Model file for the job. Use its own axes, mm. Face numbers are marked on the shaded views. A direction names the side the tool comes from. Give positions to 0.01 mm unless a question says otherwise; leave off trailing zeros. Loops run counter-clockwise (first coordinate to the right, second up) from the corner with the lowest first, then second, coordinate; pieces in that order, holes last. Notation, with made-up numbers: (45, -3.5) - (63, -3.5) arc R19 cw to (63, 2.5) - close; hole circle Ø3 at (-39, -15). An arc over 180 degrees is marked (long way). Answer as CSV lines item,"result". Start each with the question number.
Item 1: Drill centre lines: L1, parallel to Y at x = 0, z = 2.45; L2, parallel to Y at x = -1.25, z = 1.55; L3, parallel to X at y = 6, z = 2.25. Where is each one in solid material? Low to high. Write a range as from..to.
Item 2: Tool access for the marked faces 1 and 2: list every direction of +Z, -Z, +X, -X, +Y, -Y with a clear straight run to the whole face (end or side of a thin tool).
Item 3: Saw through at C-C on z = 1.1. Give the cut face in (x, y), plus the area to 3 significant figures.
Item 4: Saw through at B-B on x = 1. Give the cut face in (y, z), plus the area to 3 significant figures.
Item 5: Pin check, flat tips, straight feed: pin 1 (7 mm diameter, centred on x = 0, y = -25, fed in from -Z); pin 2 (2 mm diameter, centred on x = -4, z = 4, fed in from +Y); pin 3 (1 mm diameter, centred on x = 5, z = 3.5, fed in from -Y). Stop position of each tip, or through.
Item 6: Pull direction Y, two halves, no side cores. Call the marked faces 3, 4, 5 and 6: pulls with the +Y half, pulls with the -Y half, needs draft (parallel to the pull), parting line crosses it, or undercut.
Item 7: Saw through at D-D on y = 24. Give the cut face in (x, z).
Item 8: Saw through at A-A on y = 8. Give the cut face in (x, z), plus the area to 3 significant figures.
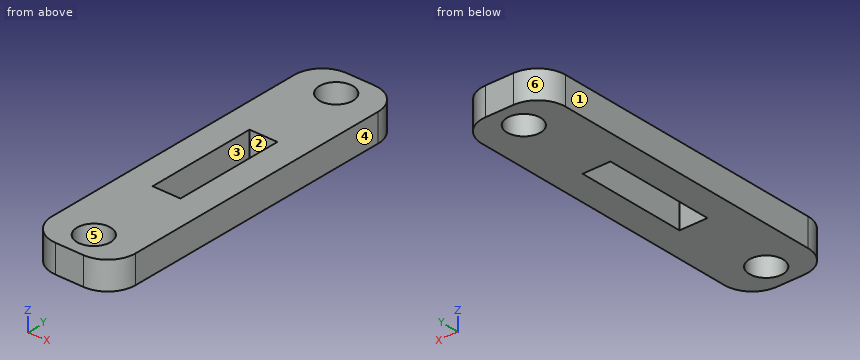
from build123d import *

# Parameters (mm, degrees)
F0_W     = 15
F0_H     = 60
F1_DEPTH = 5
F2_R     = 5
F4_W     = 5
F4_H     = 20
F5_DEPTH = 5
F3_R     = 3
F6_DEPTH = 5


with BuildPart() as f1:
    # F0 (on Top) → F1 (new body)
    with BuildSketch(Plane.XY):
        Rectangle(F0_W, F0_H)
    extrude(amount=F1_DEPTH)

    # F2
    f2_edges = [f1.edges().sort_by_distance(p)[0] for p in [
        (7.5, -30, 2.5),
        (-7.5, -30, 2.5),
        (7.5, 30, 2.5),
        (-7.5, 30, 2.5),
    ]]
    fillet(f2_edges, radius=F2_R)

    # F4 (on face) → F5 (cut, through all)
    with BuildSketch(Plane.XY.offset(5)):
        Rectangle(F4_W, F4_H)
    extrude(amount=-F5_DEPTH, mode=Mode.SUBTRACT)

    # F3 (on face) → F6 (cut, through all)
    with BuildSketch(Plane.XY.offset(5)):
        with Locations((0, -25)):
            Circle(F3_R)
        with Locations((0, 25)):
            Circle(F3_R)
    extrude(amount=-F6_DEPTH, mode=Mode.SUBTRACT)


solid = f1.part
Responses:
1,L1,"-30..-28, -22..-10, 10..22, 28..30"
1,L2,"-30..-27.73, -22.27..-10, 10..22.27, 27.73..30"
1,L3,"-7.5..-2.5, 2.5..7.5"
2,face 1,"+Z, -Z, -X, +Y, -Y"
2,face 2,"+Z, -Z"
3,outline,"(-7.5, -25) arc R5 ccw to (-2.5, -30) - (2.5, -30) arc R5 ccw to (7.5, -25) - (7.5, 25) arc R5 ccw to (2.5, 30) - (-2.5, 30) arc R5 ccw to (-7.5, 25) - close; hole circle Ø6 at (0, -25); hole circle Ø6 at (0, 25); hole (-2.5, -10) - (2.5, -10) - (2.5, 10) - (-2.5, 10) - close"
3,area,"722 mm2"
4,outline,"(-30, 0) - (-27.83, 0) - (-27.83, 5) - (-30, 5) - close; (-22.17, 0) - (-10, 0) - (-10, 5) - (-22.17, 5) - close; (10, 0) - (22.17, 0) - (22.17, 5) - (10, 5) - close; (27.83, 0) - (30, 0) - (30, 5) - (27.83, 5) - close"
4,area,"143 mm2"
5,pin 1,"z = 0"
5,pin 2,"y = 29.97"
5,pin 3,"y = -29.58"
6,face 3,"undercut"
6,face 4,"needs draft"
6,face 5,"undercut"
6,face 6,"pulls with the +Y half"
7,outline,"(-7.5, 0) - (-2.83, 0) - (-2.83, 5) - (-7.5, 5) - close; (2.83, 0) - (7.5, 0) - (7.5, 5) - (2.83, 5) - close"
8,outline,"(-7.5, 0) - (-2.5, 0) - (-2.5, 5) - (-7.5, 5) - close; (2.5, 0) - (7.5, 0) - (7.5, 5) - (2.5, 5) - close"
8,area,"50.0 mm2"
